Read the model definition and answer for the solid it produces. Units are mm, in the model's axes. Face numbers are marked on the shaded views. A direction names the side the tool comes from. Round coordinates to 2 decimals unless told otherwise and drop trailing zeros. Answer as CSV lines item,"result".
Autodesk Inventor part; units mm, degrees
ref_plane "rot_XY" through (0, 6.6675, 0) normal (1, 0, 0) x (0, 0, -1)
ref_plane "rot_YZ" through (0, 6.6675, 0) normal (0, 0, -1) x (0, 1, 0)
ref_plane "rot_ZX" through (0, 6.6675, 0) normal (0, 1, 0) x (1, 0, 0)
sketch "Sketch_2" plane through (0, -0.254, 0) normal (0, 1, 0) x (1, 0, 0)
  line L0 (-3.9497, -5.1435) -> (-3.9497, -6.3724)
  arc A0 (-3.9497, -6.3724) -> (-3.8197, -6.5024) centre (-3.8197, -6.3724) ccw
  line L1 (-3.8197, -6.5024) -> (3.8197, -6.5024)
  arc A1 (3.8197, -6.5024) -> (3.9497, -6.3724) centre (3.8197, -6.3724) ccw
  line L2 (3.9497, -6.3724) -> (3.9497, -5.1435)
  line L3 (3.9497, -5.1435) -> (3.6957, -5.1435)
  line L4 (3.6957, -5.1435) -> (3.6957, -2.9397)
  line L5 (3.6957, -2.9397) -> (3.3147, -2.8725)
  line L6 (3.3147, -2.8725) -> (3.3147, -1.8265)
  line L7 (3.3147, -1.8265) -> (3.6957, -1.7593)
  line L8 (3.6957, -1.7593) -> (3.6957, 1.7593)
  line L9 (3.6957, 1.7593) -> (3.3147, 1.8265)
  line L10 (3.3147, 1.8265) -> (3.3147, 2.8725)
  line L11 (3.3147, 2.8725) -> (3.6957, 2.9397)
  line L12 (3.6957, 2.9397) -> (3.6957, 5.1435)
  line L13 (3.6957, 5.1435) -> (3.9497, 5.1435)
  line L14 (3.9497, 5.1435) -> (3.9497, 6.3724)
  arc A2 (3.9497, 6.3724) -> (3.8197, 6.5024) centre (3.8197, 6.3724) ccw
  line L15 (3.8197, 6.5024) -> (-3.8197, 6.5024)
  arc A3 (-3.8197, 6.5024) -> (-3.9497, 6.3724) centre (-3.8197, 6.3724) ccw
  line L16 (-3.9497, 6.3724) -> (-3.9497, 5.1435)
  line L17 (-3.9497, 5.1435) -> (-3.6957, 5.1435)
  line L18 (-3.6957, 5.1435) -> (-3.6957, 2.9397)
  line L19 (-3.6957, 2.9397) -> (-3.3147, 2.8725)
  line L20 (-3.3147, 2.8725) -> (-3.3147, 1.8265)
  line L21 (-3.3147, 1.8265) -> (-3.6957, 1.7593)
  line L22 (-3.6957, 1.7593) -> (-3.6957, -1.7593)
  line L23 (-3.6957, -1.7593) -> (-3.3147, -1.8265)
  line L24 (-3.3147, -1.8265) -> (-3.3147, -2.8725)
  line L25 (-3.3147, -2.8725) -> (-3.6957, -2.9397)
  line L26 (-3.6957, -2.9397) -> (-3.6957, -5.1435)
  line L27 (-3.6957, -5.1435) -> (-3.9497, -5.1435)
extrude "Extrusion1" add sketch "Sketch_2" against normal blind 9.1694
sketch "Sketch_1" plane through (0, -9.4234, 0) normal (0, 1, 0) x (1, 0, 0)
  line L0 (-3.1877, 6.1184) -> (-3.1877, -6.1184)
  arc A0 (-3.1877, -6.1184) -> (-3.0577, -6.2484) centre (-3.0577, -6.1184) ccw
  line L1 (-3.0577, -6.2484) -> (3.0577, -6.2484)
  arc A1 (3.0577, -6.2484) -> (3.1877, -6.1184) centre (3.0577, -6.1184) ccw
  line L2 (3.1877, -6.1184) -> (3.1877, 6.1184)
  arc A2 (3.1877, 6.1184) -> (3.0577, 6.2484) centre (3.0577, 6.1184) ccw
  line L3 (3.0577, 6.2484) -> (-3.0577, 6.2484)
  arc A3 (-3.0577, 6.2484) -> (-3.1877, 6.1184) centre (-3.0577, 6.1184) ccw
extrude "Extrusion2" cut sketch "Sketch_1" along normal blind 0.0254
sketch "Sketch_7" plane through (0, -9.4234, 0) normal (0, 1, 0) x (1, 0, 0)
  line L0 (-1.0033, 5.0927) -> (-1.0033, 4.3053)
  line L1 (-1.0033, 4.3053) -> (1.0033, 4.3053)
  line L2 (1.0033, 4.3053) -> (1.0033, 5.0927)
  line L3 (1.0033, 5.0927) -> (-1.0033, 5.0927)
extrude "Extrusion3" cut sketch "Sketch_7" along normal blind 0.254
pattern_linear "Rectangular Pattern1" count 3 spacing 4.699 along (0, 0, 1) of "Extrusion3"
ref_plane "rot_XY" through (0, 6.6675, 0) normal (1, 0, 0) x (0, 0, -1)
ref_plane "rot_YZ" through (0, 6.6675, 0) normal (0, 0, -1) x (0, 1, 0)
ref_plane "rot_ZX" through (0, 6.6675, 0) normal (0, 1, 0) x (1, 0, 0)
ref_plane "to_cover_XY" through (0, -0.254, 0) normal (0, 1, 0) x (1, 0, 0)
ref_plane "to_cover_YZ" through (0, -0.254, 0) normal (1, 0, 0) x (0, 0, -1)
ref_plane "to_cover_ZX" through (0, -0.254, 0) normal (0, 0, -1) x (0, 1, 0)
ref_plane "to_terminals_XY" through (0, -9.4234, 0) normal (0, 1, 0) x (1, 0, 0)
ref_plane "to_terminals_YZ" through (0, -9.4234, 0) normal (1, 0, 0) x (0, 0, -1)
ref_plane "to_terminals_ZX" through (0, -9.4234, 0) normal (0, 0, -1) x (0, 1, 0)
properties part number "M20191SS1W01-switch"
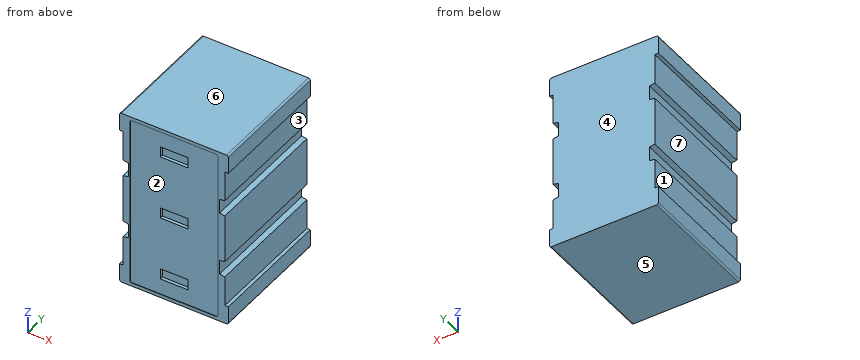
1) Each of these flat-tipped pins is pushed along its axis until it touches: P1, Ø3, axis at y = -5, z = 1, coming from the +X side; P2, Ø1.5, axis at x = -1, z = 2, coming from the -Y side; P3, Ø1.1, axis at y = -5.5, z = -4.5, coming from the -X side. Where does it stop, or does it pass through?
Evaluation:
P1,"stops at x = 3.7"
P2,"stops at y = -9.4"
P3,"stops at x = -3.7"
2) Straight lines are drawn through the part: line 1 (Z direction, x = 3.75, y = -5.25); line 2 (Z direction, x = 3.5, y = -1.25); line 3 (X direction, y = -1.25, z = 1.25). For each, find the intervals that lie inside material, in ascending order.
Evaluation:
line 1,"z = -6.5 to -5.14, 5.14 to 6.5"
line 2,"z = -6.5 to -2.91, -1.79 to 1.79, 2.91 to 6.5"
line 3,"x = -3.7 to 3.7"
3) Determine the mould class of the marked faces 5, 6 and 7 for opening direction Z: released by +Z, released by -Z, zero draft, split by the parting line, or undercut.
Evaluation:
face 5,"released by -Z"
face 6,"released by +Z"
face 7,"undercut"
4) A tool of negligible diameter and unlimited length cuts with its end or side. For the marked faces 1, 2, 3 and 4, from which of +Z, -Z, +X, -X, +Y, -Y can it reach the whole face along a straight path? Write none if from no direction.
Evaluation:
face 1,"-X, +Y, -Y"
face 2,"-Y"
face 3,"+X, +Y, -Y"
face 4,"+Z, -Z, +X, -X, +Y"
